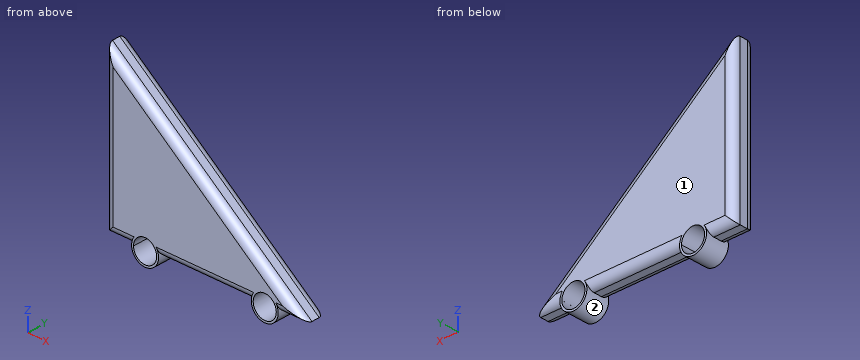
from build123d import *

# Parameters (mm, degrees)
F1_DEPTH = 15
F2_R     = 5
F3_R     = 5
F4_T     = -2.5


with BuildPart() as f1:
    # F0 (on Front) → F1 (new body)
    with BuildSketch(Plane.XZ):
        with BuildLine():
            Line((56.7000245671, -51.0693943679), (-70.2999754329, 50.5306056321))
            Line((-70.2999754329, 50.5306056321), (-70.2999754329, -51.0693943679))
            Line((-70.2999754329, -51.0693943679), (-53.4999754329, -51.0693943679))
            ThreePointArc((-53.4999754329, -51.0693943679), (-44.8999754329, -42.4693943679), (-36.2999754329, -51.0693943679))
            Line((-36.2999754329, -51.0693943679), (22.7000245671, -51.0693943679))
            ThreePointArc((22.7000245671, -51.0693943679), (31.3000245671, -42.4693943679), (39.9000245671, -51.0693943679))
            Line((39.9000245671, -51.0693943679), (56.7000245671, -51.0693943679))
        make_face()
        with BuildLine():
            ThreePointArc((-36.2999754329, -51.0693943679), (-44.8999754329, -42.4693943679), (-53.4999754329, -51.0693943679))
            ThreePointArc((-53.4999754329, -51.0693943679), (-44.8999754329, -59.6557734847), (-36.2999754329, -51.0693943679))
        make_face()
        with BuildLine():
            ThreePointArc((-37.5524947041, -51.0557626811), (-44.8931595866, -58.4032402486), (-52.2474435165, -51.0693943679))
            ThreePointArc((-52.2474435165, -51.0693943679), (-44.9067912793, -43.7082851136), (-37.5524947041, -51.0557626811))
        make_face(mode=Mode.SUBTRACT)
        with BuildLine():
            ThreePointArc((22.7000245671, -51.0693943679), (31.3000245671, -59.6537478643), (39.9000245671, -51.0693943679))
            ThreePointArc((39.9000245671, -51.0693943679), (31.3000245671, -42.4693943679), (22.7000245671, -51.0693943679))
        make_face()
        with BuildLine():
            ThreePointArc((38.6475245671, -51.053733605), (38.6475203945, -51.0615639909), (38.647507877, -51.0693943679))
            ThreePointArc((38.647507877, -51.0693943679), (23.9525287396, -51.0459032191), (38.6475245671, -51.053733605))
        make_face(mode=Mode.SUBTRACT)
    extrude(amount=F1_DEPTH)

    # F2
    f2_edges = [f1.edges().sort_by_distance(p)[0] for p in [
        (-70.299975, -15, -0.269394),
        (-6.799975, -15, -0.269394),
        (-6.799975, -15, -51.069394),
        (-61.899975, -15, -51.069394),
        (48.300025, -15, -51.069394),
    ]]
    fillet(f2_edges, radius=F2_R)

    # F3
    f3_edges = [f1.edges().sort_by_distance(p)[0] for p in [
        (-6.799975, 0, -0.269394),
        (-6.799975, 0, -51.069394),
        (48.300025, 0, -51.069394),
        (-70.299975, 0, -0.269394),
        (-61.899975, 0, -51.069394),
    ]]
    fillet(f3_edges, radius=F3_R)

    # F4 (hollow: no face is removed)
    offset(amount=F4_T, mode=Mode.SUBTRACT)


solid = f1.part
Build history of the part. All positions in model axes, mm. Face numbers are marked on the shaded views. Give positions to 0.01 mm unless a question says otherwise; leave off trailing zeros. Use one line per item in the form item = value. Start each with the question number.
1. Band-saw the part on A-A on y = -8.5. Count the separate pieces of the cut face and the enclosed holes in it, plus the area to 3 significant figures.
2. Drop flat-ended pins along their axis: pin 1 Ø5 at (y, z) = (-10, 12.5) entering from +X; pin 2 Ø3 at (x, y) = (-12.5, -10.5) entering from -Z; pin 3 Ø3 at (x, y) = (20, -3) entering from +Z; pin 4 Ø9 at (x, z) = (31.3, -51.05) entering from -Y. Give the stop position or say it passes through.
3. Two-plate mould, pull along X, no slides. Class the marked faces 1 and 2: released by +X, released by -X, zero draft, split by the parting line, or undercut.
4. Probe line 1 (Y direction, x = 3, z = -32); line 2 (Z direction, x = 26, y = -7.5); line 3 (X direction, y = -5.75, z = 10.5). List the from-to ranges inside material, lowest first. Write a range as [from, to].
Conclusion:
q1.separate_pieces = 1
q1.enclosed_holes = 3
q1.area = 1,040 mm²
q2.pin_1 = -19.64
q2.pin_2 = -51.07
q2.pin_3 = -20.87
q2.pin_4 = through
q3.face_1 = zero draft
q3.face_2 = undercut
q4.line_1 = [-15, -12.5], [-2.5, 0]
q4.line_2 = [-57.83, -56.14], [-45.96, -42.75], [-29.71, -26.51]
q4.line_3 = [-70.3, -67.8], [-24.26, -20.26]
